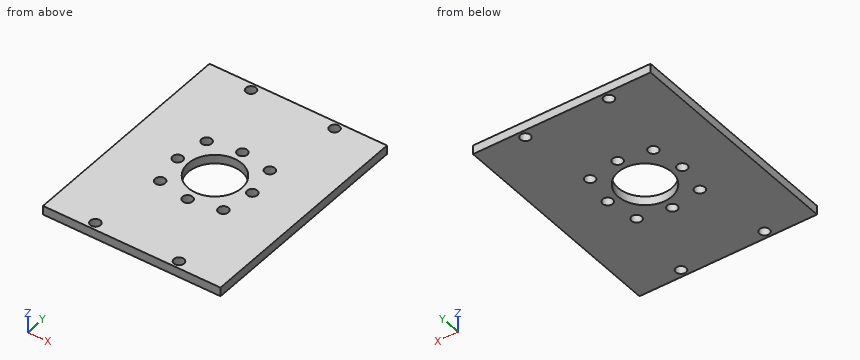
Autodesk Fusion 360 part; units mm, degrees
sketch "Sketch1" plane through (0, 0, 0) normal (0, 0, 1) x (1, 0, 0)
  circle A0 centre (0, 0) radius 29.75
  circle A1 centre (0, 0) radius 12.5
  circle A2 centre (0, 0) radius 15
  circle A3 centre (0, 12.5) radius 1.7
  circle A4 centre (-10.6066, 10.6066) radius 1.7
  circle A5 centre (-10.6066, -10.6066) radius 1.7
  circle A6 centre (-12.5, 0) radius 1.7
  circle A7 centre (10.6066, -10.6066) radius 1.7
  circle A8 centre (0, -12.5) radius 1.7
  circle A9 centre (10.6066, 10.6066) radius 1.7
  circle A10 centre (12.5, 0) radius 1.7
  circle A11 centre (-14, 35.5) radius 1.7
  circle A12 centre (14, 35.5) radius 1.7
  circle A13 centre (14, -35.5) radius 1.7
  circle A14 centre (-14, -35.5) radius 1.7
  line L0 (-29.75, 38) -> (29.75, 38)
  line L1 (29.75, 38) -> (29.75, -38)
  line L2 (29.75, -38) -> (-29.75, -38)
  line L3 (-29.75, -38) -> (-29.75, 38)
  circle A15 centre (0, 0) radius 9
  dimension "d1" = 59.5
  dimension "d2" = 25
  dimension "d3" = 30
  dimension "d5" = 3.4
  dimension "d10" = 360
  dimension "d13" = 3.4
  dimension "d14" = 3.4
  dimension "d15" = 3.4
  dimension "d16" = 3.4
  dimension "d17" = 59.5
  dimension "d18" = 76
  dimension "d19" = 18
extrude "Extrude1" add sketch "Sketch1" along normal blind 3 contours A0 | A0 L1 L2 L3 | A0 L0 L1 L3 | A1 A3 A6 A8 A10 | A2 A4 A5 A7 A9
Read the model definition and answer for the solid it produces. Units are mm, in the model's axes. Coordinates: 2 decimals unless noted, no trailing zeros. Order: outer loops, then holes, each group sorted by start corner. A loop starts at its lowest first (then second) coordinate and runs counter-clockwise, first axis right, second up. Notation, with made-up numbers: (15, 71) - (25, 71) arc R19 ccw to (25, 104) - close; hole circle Ø5 at (58.25, -9.75). An arc over 180 degrees is marked (long way). Answer as a JSON object with one key per item and string values. Group by question number.
Item 1: Section B-B (y = 0) is taken. Give the vertices of the cut face in (x, z), plus the area to 3 significant figures.
Item 2: Section D-D (z = 2.2) is taken. State how many separate pieces and enclosed holes the cut face has, plus the area to 3 significant figures.
Item 3: Section A-A (x = 0) is taken. Give the vertices of the cut face in (y, z).
Item 4: Consider probe 1 along Y at (x, z) = (0, 1.85); probe 2 along Y at (x, z) = (-10.5, 1.1); probe 3 along X at (y, z) = (11.5, 1.85). Determine where each line is inside the solid, lowest interval first. Write a range as from..to.
Item 5: Section C-C (y = -35.5) is taken. Give the vertices of the cut face in (x, z), plus the area to 3 significant figures.
Results are:
{
 "1": {"outline": "(-29.75, 0) - (-14.2, 0) - (-14.2, 3) - (-29.75, 3) - close; (-10.8, 0) - (-9, 0) - (-9, 3) - (-10.8, 3) - close; (9, 0) - (10.8, 0) - (10.8, 3) - (9, 3) - close; (14.2, 0) - (29.75, 0) - (29.75, 3) - (14.2, 3) - close", "area": "104 mm^2"},
 "2": {"separate pieces": "1", "enclosed holes": "13", "area": "4,160 mm^2"},
 "3": {"outline": "(-38, 0) - (-14.2, 0) - (-14.2, 3) - (-38, 3) - close; (-10.8, 0) - (-9, 0) - (-9, 3) - (-10.8, 3) - close; (9, 0) - (10.8, 0) - (10.8, 3) - (9, 3) - close; (14.2, 0) - (38, 0) - (38, 3) - (14.2, 3) - close"},
 "4": {"probe 1": "y = -38..-14.2, -10.8..-9, 9..10.8, 14.2..38", "probe 2": "y = -38..-12.3, -8.91..8.91, 12.3..38", "probe 3": "x = -29.75..-12.05, -9.16..-1.37, 1.37..9.16, 12.05..29.75"},
 "5": {"outline": "(-29.75, 0) - (-15.7, 0) - (-15.7, 3) - (-29.75, 3) - close; (-12.3, 0) - (12.3, 0) - (12.3, 3) - (-12.3, 3) - close; (15.7, 0) - (29.75, 0) - (29.75, 3) - (15.7, 3) - close", "area": "158 mm^2"}
}
